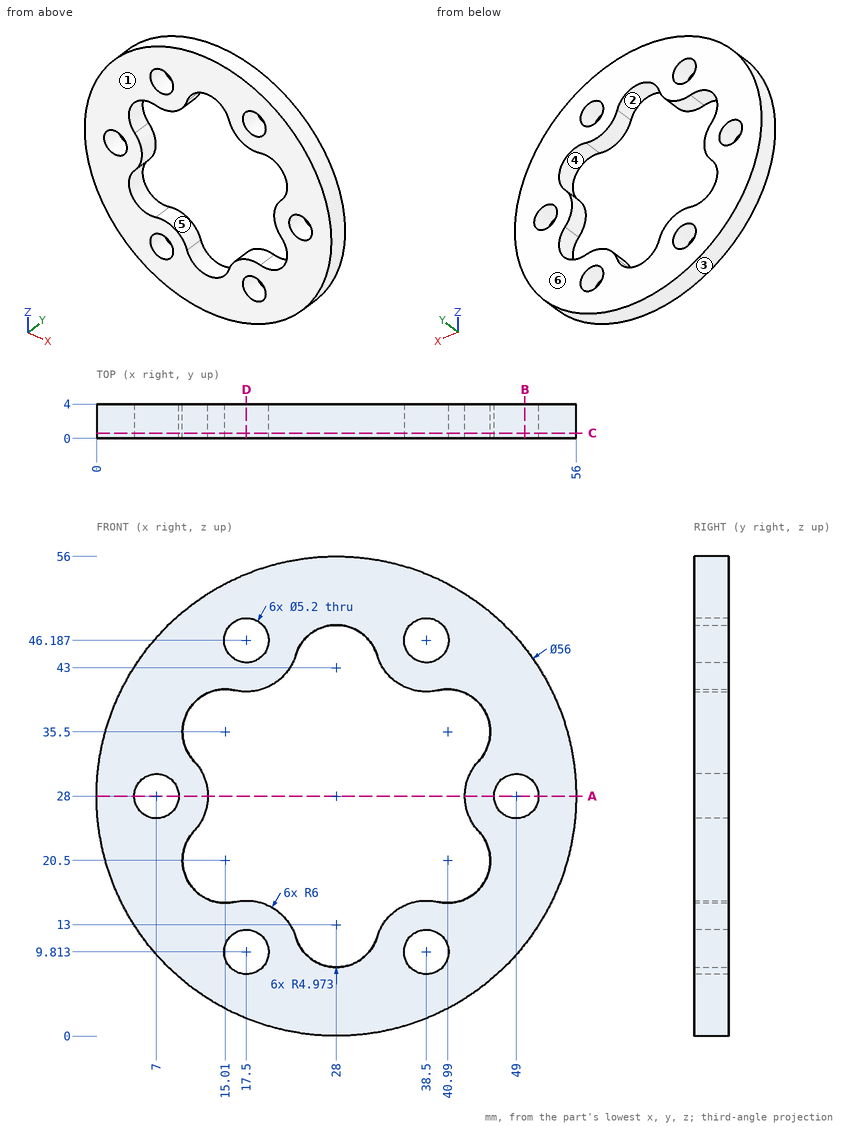
The drawing under review shows one solid part. Ordinate dimensions are in mm from its lowest x, y, z. A direction names the side the tool comes from. Give positions to 0.01 mm unless a question says otherwise; leave off trailing zeros. Write each loop counter-clockwise with the first axis right and the second up, starting at its lowest first coordinate (ties: lowest second). Pieces come first, ordered by that corner, then holes.
1. Wall thickness on L1, parallel to X at y = 0.8, z = 28; L2, parallel to Z at x = 17.5, y = 2 (1 decimal); L3, parallel to Z at x = 12.5, y = 1.2 (1 decimal): over which ranges is each line inside the solid? List them lowest first.
2. Add section D-D, the plane x = 17.5. Write out the cut boundary in (y, z).
3. Add section B-B, the plane x = 50. Write out the cut boundary in (y, z), plus the area to 3 significant figures.
4. Add section C-C, the plane y = 0.6. Write out the cut boundary in (x, z) (1 decimal), plus the area to 3 significant figures.
5. For P1, Ø2, axis at x = 13, y = 1, coming from the -Z side; P2, Ø4, axis at x = 7, z = 28, coming from the +Y side; P3, Ø1.5, axis at x = 30.5, y = 1.5, coming from the +Z side (1 decimal), all flat-tipped, find the tip position at first contact; note any pin that passes through.
6. Add section A-A, the plane z = 28. Write out the cut boundary in (x, y).
7. Draft analysis for pull direction X (two halves, no side actions). For the marked faces 3, 4, 5 and 6, state which applies: +X half, -X half, draft (parallel to the pull), parting line (faces both ways), or undercut.
8. Tool access review of the marked faces 1 and 2: name each direction out of +Z, -Z, +X, -X, +Y, -Y from which nothing blocks a thin tool from reaching the whole face with its end or side.
Worked answers:
1. L1: x = 0 to 4.4, 9.6 to 13, 43 to 46.4, 51.6 to 56
1. L2: z = 2 to 7.2, 12.4 to 15.8, 40.2 to 43.6, 48.8 to 54
1. L3: z = 4.7 to 16.2, 25.6 to 30.4, 39.8 to 51.3
2. outline: (0, 2.04) - (4, 2.04) - (4, 7.21) - (0, 7.21) - close; (0, 12.41) - (4, 12.41) - (4, 15.81) - (0, 15.81) - close; (0, 40.19) - (4, 40.19) - (4, 43.59) - (0, 43.59) - close; (0, 48.79) - (4, 48.79) - (4, 53.96) - (0, 53.96) - close
3. outline: (0, 10.68) - (4, 10.68) - (4, 25.6) - (0, 25.6) - close; (0, 30.4) - (4, 30.4) - (4, 45.32) - (0, 45.32) - close
3. area: 119 mm2
4. outline: circle Ø56 at (28, 28); hole circle Ø5.2 at (7, 28); hole (11.4, 23.9) arc R5 ccw to (16.1, 15.7) arc R6 cw to (23.2, 11.6) arc R5 ccw to (32.8, 11.6) arc R6 cw to (39.9, 15.7) arc R5 ccw to (44.6, 23.9) arc R6 cw to (44.6, 32.1) arc R5 ccw to (39.9, 40.3) arc R6 cw to (32.8, 44.4) arc R5 ccw to (23.2, 44.4) arc R6 cw to (16.1, 40.3) arc R5 ccw to (11.4, 32.1) arc R6 cw to start; hole circle Ø5.2 at (17.5, 9.8); hole circle Ø5.2 at (17.5, 46.2); hole circle Ø5.2 at (38.5, 9.8); hole circle Ø5.2 at (38.5, 46.2); hole circle Ø5.2 at (49, 28)
4. area: 1,360 mm2
5. P1: stops at z = 3.75
5. P2: passes through
5. P3: stops at z = 55.9
6. outline: (0, 0) - (4.4, 0) - (4.4, 4) - (0, 4) - close; (9.6, 0) - (13, 0) - (13, 4) - (9.6, 4) - close; (43, 0) - (46.4, 0) - (46.4, 4) - (43, 4) - close; (51.6, 0) - (56, 0) - (56, 4) - (51.6, 4) - close
7. face 3: parting line
7. face 4: undercut
7. face 5: undercut
7. face 6: draft
8. face 1: +Z, -Z, +X, -X, -Y
8. face 2: +Y, -Y
